from build123d import *

# Parameters (mm, degrees)
SKETCH1_W             = 30
SKETCH1_H             = 50
BOSS_EXTRUDE1_DEPTH   = 6
M5X0_8_TAPPED_HOLE1_D = 4.2
CHAMFER1_SIZE         = 2


with BuildPart() as part:
    # Sketch1 → Boss-Extrude1 (new body)
    with BuildSketch(Plane.XY):
        with Locations((15, 0)):
            Rectangle(SKETCH1_W, SKETCH1_H)
    extrude(amount=BOSS_EXTRUDE1_DEPTH)

    # M5x0.8 Tapped Hole1 (through all)
    with Locations(Plane.XY.offset(6)):
        with Locations((6, 18.7), (6, -18.7), (24, -18.7), (24, 18.7)):
            Hole(M5X0_8_TAPPED_HOLE1_D / 2)

    # Chamfer1
    chamfer1_edges = [part.edges().sort_by_distance(p)[0] for p in [
        (0, 25, 3),
        (30, 25, 3),
        (30, -25, 3),
        (0, -25, 3),
    ]]
    chamfer(chamfer1_edges, length=CHAMFER1_SIZE)


solid = part.part
CAD build for the part. Positions are in the model's coordinates, mm. Round coordinates to 2 decimals unless told otherwise and drop trailing zeros. Order: outer loops, then holes, each group sorted by start corner. A loop starts at its lowest first (then second) coordinate and runs counter-clockwise, first axis right, second up. Notation, with made-up numbers: M -24,-12 L 0,-12 A14 cw 0,0 Z; hole C 70,79 d9. An arc over 180 degrees is marked long. Use one line per item in the form item = value.
Q1. Saw through at A-A on x = 24. Give the cut face in (y, z).
Recorded:
outline = M -25,0 L -20.8,0 L -20.8,6 L -25,6 Z; M -16.6,0 L 16.6,0 L 16.6,6 L -16.6,6 Z; M 20.8,0 L 25,0 L 25,6 L 20.8,6 Z
Q2. Saw through at C-C on z = 2.05. Give the cut face in (x, y).
Recorded:
outline = M 0,-23 L 2,-25 L 28,-25 L 30,-23 L 30,23 L 28,25 L 2,25 L 0,23 Z; hole C 6,-18.7 d4.2; hole C 6,18.7 d4.2; hole C 24,-18.7 d4.2; hole C 24,18.7 d4.2
Q3. Flat gauge pin, fed straight in: P1, Ø12, axis at x = 26.5, y = 10.5, coming from the -Z side. Where does the tip first touch, or does it go through?
Recorded:
P1 = 0
Q4. Two-plate mould, pull along X, no slides. Class faces 1 (the flat face through (30, 0, 3)), 2 (the flat face through (0, 0, 3)), 3 (the cylindrical face through (21.997, 19.331, 2.958)), 4 (the cylindrical face through (4.87, 20.47, 2.96)): +X half, -X half, draft (parallel to the pull), parting line (faces both ways), or undercut.
Recorded:
face_1 = +X half
face_2 = -X half
face_3 = undercut
face_4 = undercut
Q5. Saw through at B-B on y = 18.7. Give the cut face in (x, z), then the cut area to 3 significant figures.
Recorded:
outline = M 0,0 L 3.9,0 L 3.9,6 L 0,6 Z; M 8.1,0 L 21.9,0 L 21.9,6 L 8.1,6 Z; M 26.1,0 L 30,0 L 30,6 L 26.1,6 Z
area = 130 mm^2
Q6. Probe L1, parallel to Y at x = 6, z = 3.4; L2, parallel to X at y = -20.5, z = 1.8; L3, parallel to X at y = -17.5, z = 2.9. List the from-to ranges inside material, lowest first.
Recorded:
L1 = -25 to -20.8, -16.6 to 16.6, 20.8 to 25
L2 = 0 to 4.92, 7.08 to 22.92, 25.08 to 30
L3 = 0 to 4.28, 7.72 to 22.28, 25.72 to 30
